```python
from build123d import *

# Parameters (mm, degrees)
F0_R      = 25
F1_DEPTH  = 20
F2_R      = 19.99999
F3_R      = 5
F4_R      = 20.4165647278
F5_DEPTH  = 10
F6_R      = 26.9213297652
F7_DEPTH  = 10
F8_R      = 19.8358108325
F9_DEPTH  = 5
F10_R     = 2
F11_R     = 7.5
F12_DEPTH = 50


# Not quite as in the source:
# - a fillet or chamfer is up to 0.001 mm smaller than in the source, because OpenCascade refuses the exact size


with BuildPart() as f1:
    # F0 (on Right) → F1 (new body)
    with BuildSketch(Plane.YZ):
        Circle(F0_R)
    extrude(amount=F1_DEPTH)

    # F2 (radius 20 in the source; OpenCascade refuses exactly that, so slightly less here)
    f2_edges = [f1.edges().sort_by_distance(p)[0] for p in [
        (0, -25, 0),
    ]]
    fillet(f2_edges, radius=F2_R)

    # F3
    f3_edges = [f1.edges().sort_by_distance(p)[0] for p in [
        (20, -25, 0),
    ]]
    fillet(f3_edges, radius=F3_R)

    # F4 (on face) → F5 (join)
    with BuildSketch(Plane.YZ.offset(20)):
        Circle(F4_R)
    extrude(amount=F5_DEPTH)

    # F6 (on face) → F7 (join)
    with BuildSketch(Plane.YZ.offset(30)):
        Circle(F6_R)
    extrude(amount=F7_DEPTH)

    # F8 (on face) → F9 (join)
    with BuildSketch(Plane.YZ.offset(40)):
        Circle(F8_R)
    extrude(amount=F9_DEPTH)

    # F10
    f10_edges = [f1.edges().sort_by_distance(p)[0] for p in [
        (45, -19.835811, 0),
    ]]
    fillet(f10_edges, radius=F10_R)

    # F11 (on face) → F12 (join)
    with BuildSketch(Plane.YZ.offset(45)):
        Circle(F11_R)
    extrude(amount=F12_DEPTH)


solid = f1.part
```
Can you work these out from the model? Positions are in its coordinate system, mm. A direction names the side the tool comes from. Coordinates: 2 decimals unless noted, no trailing zeros. Write each loop counter-clockwise with the first axis right and the second up, starting at its lowest first coordinate (ties: lowest second). Pieces come first, ordered by that corner, then holes. Notation, with made-up numbers: (-8, 52.25) - (41, 52.25) arc R3 cw to (41, 56.25) - close; hole circle Ø6 at (21.25, 15). An arc over 180 degrees is marked (long way). Return JSON: item names as keys, results as strings.
Q1. Thinking about a two-plate mould opening in X: for faces 4 (the flat face through (45, 0, -8)), 5 (the cylindrical face through (69.65, -7.493, 0.33)), 6 (the flat face through (30, 10, 18)), which applies, +X half, -X half, draft (parallel to the pull), parting line (faces both ways), or undercut?
Computed values:
{"face 4": "+X half", "face 5": "draft", "face 6": "undercut"}
Q2. I'm going to push flat-ended pins straight in: pin 1 Ø10 at (x, z) = (64.5, -5.5) entering from +Y; pin 2 Ø5 at (y, z) = (-8.5, -4) entering from -X; pin 3 Ø2 at (x, y) = (9.5, 15.5) entering from -Z. Where does each tip first touch, or does it pass through?
Computed values:
{"pin 1": "stops at y = 7.48", "pin 2": "stops at x = 0.09", "pin 3": "stops at z = -16.88"}
Q3. Please list where these lines run through material, in increasing order: L1, parallel to X at y = 14.5, z = -18.5; L2, parallel to X at y = -23.5, z = -10.5; L3, parallel to X at y = 11, z = 8.5. Write a range as from..to.
Computed values:
{"L1": "x = 12.41..17.44, 30..40", "L2": "x = 30..40", "L3": "x = 2.09..45"}
Q4. On a 3-axis mill with a long thin cutter (end or side, diameter ignored), from which of +Z, -Z, +X, -X, +Y, -Y can I reach the whole of each face in a straight line? I mean faces 1 (the cylindrical face through (24.93, -16.202, -12.423)), 2 (the cylindrical face through (41.479, -4.3, -19.364)), 3 (the flat face through (95, 0, 0)). Say none if no direction works.
Computed values:
{"face 1": "none", "face 2": "+X", "face 3": "+Z, -Z, +X, +Y, -Y"}
Q5. If we section it at A-A (x = 42): Please give me the cut outline in (y, z).
Computed values:
{"outline": "circle Ø39.67 at (0, 0)"}
Q6. If we section it at B-B (x = 57): Please give me the cut outline in (y, z).
Computed values:
{"outline": "circle Ø15 at (0, 0)"}
